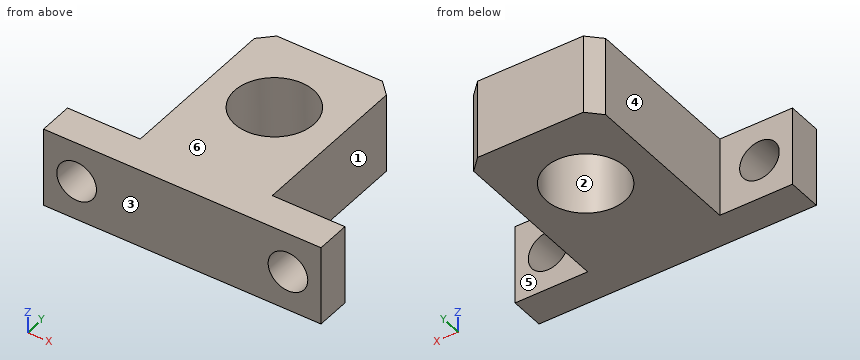
Autodesk Fusion 360 part; units mm, degrees
sketch "Boceto1" plane through (0, 0, 0) normal (0, 0, 1) x (1, 0, 0)
  line L0 (0, 0) -> (21, 0)
  line L1 (21, 0) -> (21, 5.2)
  line L2 (21, 5.2) -> (10, 5.2)
  line L3 (10, 5.2) -> (10, 30)
  line L4 (10, 30) -> (8, 32)
  line L5 (10, 30) -> (23.9079, 30) construction
  line L6 (8, 32) -> (0, 32)
  line L7 (0, 0) -> (0, 32) construction
  line L8 (-10, 30) -> (-8, 32)
  line L9 (-10, 5.2) -> (-10, 30)
  line L10 (-21, 0) -> (-21, 5.2)
  line L11 (-21, 5.2) -> (-10, 5.2)
  line L12 (-8, 32) -> (0, 32)
  circle A0 centre (0, 20) radius 6
  line L13 (0, 0) -> (-21, 0)
  dimension "d17" = 5.2
  dimension "d19" = 45
  dimension "d20" = 8
  dimension "d21" = 32
  dimension "d24" = 10
  dimension "d25" = 12
  dimension "d26" = 20
  dimension "d47" = 10
  dimension "d50" = 11
extrude "Extruir2" add sketch "Boceto1" along normal mid plane 12
sketch "Boceto7" plane through (0, 0, 0) normal (0, -1, 0) x (1, 0, 0)
  line L0 (21, -6) -> (21, 6)
  line L1 (21, 6) -> (-21, 6)
  line L2 (-21, 6) -> (-21, -6)
  line L3 (-21, -6) -> (21, -6)
  circle A0 centre (16, 0) radius 3
  circle A1 centre (-16, 0) radius 3
  dimension "d57" = 6
  dimension "d58" = 5
  dimension "d59" = 6
extrude "Extruir11" cut sketch "Boceto7" along normal mid plane 52 contours A0 | A1
extrude "Extruir6" [suppressed]
extrude "Extruir7" [suppressed]
component "Component" placed x (1, 0, 0) y (0, 1, 0) z (0, 0, 1) at (0, 0, 0)
Source: CAD feature listing. Evaluate the final solid. Frame: model axes, mm. Face numbers are marked on the shaded views. A direction names the side the tool comes from. Coordinates: 2 decimals unless noted, no trailing zeros. Loops run counter-clockwise (first coordinate to the right, second up) from the corner with the lowest first, then second, coordinate; pieces in that order, holes last. Notation, with made-up numbers: (-28, -35) - (-23, -35) arc R36 ccw to (-23, -1) - close; hole circle Ø10 at (36.5, -16.75). An arc over 180 degrees is marked (long way). One line per question, with ' | ' between items.
1) Section C-C, the plane y = 20. Return loops of the section in (x, z).
Report:
outline: (-10, -6) - (-6, -6) - (-6, 6) - (-10, 6) - close; (6, -6) - (10, -6) - (10, 6) - (6, 6) - close
2) Pull-direction query (Y, two-part tool) for the marked faces 1, 2 and 3; classes: released by +Y, released by -Y, zero draft, split by the parting line, or undercut.
Report:
face 1: zero draft | face 2: undercut | face 3: released by -Y
3) Section A-A, the plane z = 0. Return loops of the section in (x, y).
Report:
outline: (-21, 0) - (-19, 0) - (-19, 5.2) - (-21, 5.2) - close; (-13, 0) - (13, 0) - (13, 5.2) - (10, 5.2) - (10, 30) - (8, 32) - (-8, 32) - (-10, 30) - (-10, 5.2) - (-13, 5.2) - close; (19, 0) - (21, 0) - (21, 5.2) - (19, 5.2) - close; hole circle Ø12 at (0, 20)
4) Set-up query: the marked faces 4, 5 and 6. Return all of +Z, -Z, +X, -X, +Y, -Y with unobstructed straight access to the full face (end or side cutting, diameter ignored); none if empty.
Report:
face 4: +Z, -Z, -X, +Y | face 5: +Z, -Z, +X, +Y | face 6: +Z, +X, -X, +Y, -Y
5) Section B-B, the plane x = 16. Return loops of the section in (y, z).
Report:
outline: (0, -6) - (5.2, -6) - (5.2, -3) - (0, -3) - close; (0, 3) - (5.2, 3) - (5.2, 6) - (0, 6) - close
6) Section D-D, the plane y = 4. Return loops of the section in (x, z), then the cut area to 3 significant figures.
Report:
outline: (-21, -6) - (21, -6) - (21, 6) - (-21, 6) - close; hole circle Ø6 at (-16, 0); hole circle Ø6 at (16, 0) | area: 447 mm²
7) First-contact query: P1, Ø5.5, axis at x = 16, z = 0, coming from the -Y side; P2, Ø5, axis at y = 26, z = 0.5, coming from the +X side. Flat tips, straight axial feed; report the tip coordinate or a pass-through.
Report:
P1: passes through | P2: stops at x = 10
8) Line query: line 1 along Y through (x, z) = (0, 3.75); line 2 along Z through (x, y) = (16, 1.1); line 3 along Y through (x, z) = (14, 4.5). Output: solid intervals per line, ascending.
Report:
line 1: y = 0 to 14, 26 to 32 | line 2: z = -6 to -3, 3 to 6 | line 3: y = 0 to 5.2
